```python
from build123d import *

# Parameters (mm, degrees)
F1_DEPTH  = 127
F2_R      = 5.08
F3_R      = 6.35
F4_DEPTH  = 50.8
F6_W      = 10.401725
F6_H      = 2.54
F7_DEPTH  = 25.4
F5_W      = 19.589182
F5_H      = 11.334733
F8_DEPTH  = 25.4
F9_R      = 5.08
F10_W     = 12.79125
F10_H     = 9.451311
F11_DEPTH = 60


with BuildPart() as f1:
    # F0 (on Front) → F1 (new body)
    with BuildSketch(Plane.XZ):
        Polygon((0, 63.212529), (0, 0), (60.713694, 0), (60.713694, 21.285245), (44.640973, 36.063522), (69.603488, 63.212529), align=None)
    extrude(amount=F1_DEPTH)

    # F2
    f2_edges = [f1.edges().sort_by_distance(p)[0] for p in [
        (69.603488, -63.5, 63.212529),
        (60.713694, -63.5, 21.285245),
    ]]
    fillet(f2_edges, radius=F2_R)

    # F3 (on face) → F4 (cut)
    with BuildSketch(Plane.XZ.offset(127)):
        with Locations((30.356847, 22.944534)):
            Circle(F3_R)
    extrude(amount=-F4_DEPTH, mode=Mode.SUBTRACT)

    # F6 (on face) → F7 (cut)
    with BuildSketch(Plane.XZ.offset(127)):
        with Locations((18.203875, 53.85644)):
            Rectangle(F6_W, F6_H)
    extrude(amount=-F7_DEPTH, mode=Mode.SUBTRACT)

    # F5 (on face) → F8 (cut)
    with BuildSketch(Plane.XZ.offset(127)):
        with Locations((19.849312, 45.366853)):
            Rectangle(F5_W, F5_H)
    extrude(amount=-F8_DEPTH, mode=Mode.SUBTRACT)

    # F9
    f9_edges = [f1.edges().sort_by_distance(p)[0] for p in [
        (29.01582, -127, 63.212529),
    ]]
    fillet(f9_edges, radius=F9_R)

    # F10 (on face) → F11 (cut)
    with BuildSketch(Plane.XZ.offset(127)):
        with Locations((12.520159, 17.595014)):
            Rectangle(F10_W, F10_H)
    extrude(amount=-F11_DEPTH, mode=Mode.SUBTRACT)


solid = f1.part
```
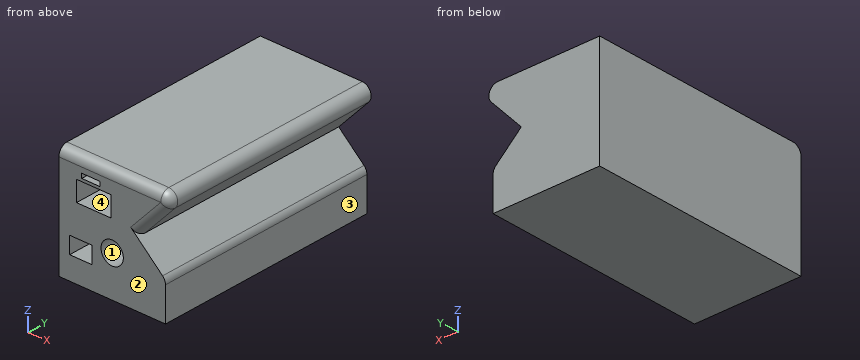
The model under review builds one solid part; all positions refer to its coordinate system, in mm. Face numbers are marked on the shaded views. Round coordinates to 2 decimals unless told otherwise and drop trailing zeros. Loops run counter-clockwise (first coordinate to the right, second up) from the corner with the lowest first, then second, coordinate; pieces in that order, holes last. Notation, with made-up numbers: (26, 50.5) - (53, 50.5) arc R14 ccw to (53, 67.5) - close; hole circle Ø8 at (-5, -34). An arc over 180 degrees is marked (long way). Write each question's results on one line, items separated by ' | '. Start each with the question number.
Q1. Take a section at C-C on y = -106. Give the boundary of the cut face in (x, z), plus the area to 3 significant figures.
Q2. Take a section at A-A on x = 8.5. Give the boundary of the cut face in (y, z).
Q3. Take a section at D-D on z = 4. Give the boundary of the cut face in (x, y), plus the area to 3 significant figures.
Q4. Wall thickness on line 1 along Z through (x, y) = (19, -113.5); line 2 along Z through (x, y) = (11, -75); line 3 along X through (y, z) = (-84, 16.5): over which ranges is each line inside the solid? List them lowest first. Write a range as [from, to].
Q5. Take a section at B-B on y = -65. Give the boundary of the cut face in (x, z), plus the area to 3 significant figures.
Q6. Insertion check: P1, Ø5.5, axis at y = -111, z = 42.5, coming from the +X side; P2, Ø1.3, axis at y = -113, z = 53.5, coming from the -X side; P3, Ø9.5, axis at y = -84.5, z = 10, coming from the +X side; P4, Ø3, axis at x = 11.5, z = 19.5, coming from the -Y side. Each pin has a flat end and moves straight along its axis. Give the tip position at first contact, or say it passes through.
Q7. Draft analysis for pull direction X (two halves, no side actions). For the marked faces 1, 2, 3 and 4, state which applies: pulls with the +X half, pulls with the -X half, needs draft (parallel to the pull), parting line crosses it, or undercut.
Data:
1) outline: (0, 0) - (60.71, 0) - (60.71, 19.06) arc R5.08 ccw to (59.07, 22.79) - (44.64, 36.06) - (61.77, 54.69) arc R5.08 ccw to (58.03, 63.21) - (0, 63.21) - close; hole (6.12, 12.87) - (18.92, 12.87) - (18.92, 22.32) - (6.12, 22.32) - close; hole (10.05, 39.7) - (29.64, 39.7) - (29.64, 51.03) - (10.05, 51.03) - close; hole (13, 52.59) - (23.4, 52.59) - (23.4, 55.13) - (13, 55.13) - close; hole circle Ø12.7 at (30.36, 22.94) | area: 3,100 mm²
2) outline: (-127, 0) - (0, 0) - (0, 63.21) - (-121.92, 63.21) arc R5.08 ccw to (-127, 58.13) - (-127, 22.32) - (-67, 22.32) - (-67, 12.87) - (-127, 12.87) - close
3) outline: (0, -127) - (60.71, -127) - (60.71, 0) - (0, 0) - close | area: 7,710 mm²
4) line 1: z = [0, 39.7], [51.03, 52.59], [55.13, 63.21] | line 2: z = [0, 12.87], [22.32, 63.21] | line 3: x = [0, 6.12], [18.92, 60.71]
5) outline: (0, 0) - (60.71, 0) - (60.71, 19.06) arc R5.08 ccw to (59.07, 22.79) - (44.64, 36.06) - (61.77, 54.69) arc R5.08 ccw to (58.03, 63.21) - (0, 63.21) - close | area: 3,590 mm²
6) P1: stops at x = 53.09 | P2: stops at x = 0 | P3: stops at x = 60.71 | P4: stops at y = -67
7) face 1: undercut | face 2: needs draft | face 3: pulls with the +X half | face 4: undercut
